For this review, take the finished solid that the model builds, in its own axes (mm). A direction names the side the tool comes from. Coordinates: 2 decimals unless noted, no trailing zeros. Write each loop counter-clockwise with the first axis right and the second up, starting at its lowest first coordinate (ties: lowest second). Pieces come first, ordered by that corner, then holes. Notation, with made-up numbers: (68, 68.5) -> (126, 68.5) arc R19 ccw to (126, 102.5) -> close; hole circle Ø2 at (0, 15.25). An arc over 180 degrees is marked (long way). One line per item, written item: value. Start each with the question number.
1) Machinability: for faces 1 (the flat face through (-44.45, 0, 0)), 2 (the cylindrical face through (42.22, 2.42, -0.1)), which of the approach directions +Z, -Z, +X, -X, +Y, -Y give a long, thin tool a straight path to every point of the face, cutting with its end or side? Answer none if there is none.
2) Add section A-A (z = -1). State the section outline as (x, y) points, and give its area (3 significant figures).
3) For probe 1 along Z at (x, y) = (39.5, 0.5); probe 2 along Z at (x, y) = (-35, 4.5); probe 3 along Y at (x, z) = (26.5, -3.5), list the stretches that pass through material, from the lowest coordinate up. Write a range as from..to.
4) Mouldability with a two-part tool opening along Z and no side actions: class faces 3 (the cylindrical face through (-0.62, -4.44, 4.54)), 4 (the cylindrical face through (0.62, -4.44, -4.54)), 5 (the cylindrical face through (47.306, -3.131, 0.223)) as released by +Z, released by -Z, zero draft, split by the parting line, or undercut.
5) For pin 1 Ø12 at (x, z) = (-21.5, -7) entering from -Y; pin 2 Ø1 at (x, z) = (-24, -4) entering from -Y; pin 3 Ø5 at (x, z) = (12.5, -6.5) entering from -Y, all flat-tipped, find the tip position at first contact; note any pin that passes through.
6) Add section C-C (y = -4). State the section outline as (x, z) points, and give its area (3 significant figures).
from build123d import *

# Parameters (mm, degrees)
F1_DEPTH = 6.35
F2_R     = 6.3499
F0_R     = 5.08
F3_DEPTH = 6.35


# Not quite as in the source:
# - a fillet or chamfer is up to 0.001 mm smaller than in the source, because OpenCascade refuses the exact size


with BuildPart() as f1:
    # F0 (on Front) → F1 (new body, symmetric)
    with BuildSketch(Plane.XZ):
        with BuildLine():
            Line((44.45, 6.35), (-44.45, 6.35))
            ThreePointArc((-44.45, 6.35), (-42.7945407024, 3.3649028089), (-42.221147458, 0))
            ThreePointArc((-42.221147458, 0), (-42.7945407024, -3.3649028089), (-44.45, -6.35))
            Line((-44.45, -6.35), (44.45, -6.35))
            ThreePointArc((44.45, -6.35), (42.221147458, 0), (44.45, 6.35))
        make_face()
        with BuildLine():
            ThreePointArc((-42.221147458, 0), (-42.7945407024, 3.3649028089), (-44.45, 6.35))
            Line((-44.45, 6.35), (-44.45, -6.35))
            ThreePointArc((-44.45, -6.35), (-42.7945407024, -3.3649028089), (-42.221147458, 0))
        make_face()
    extrude(amount=F1_DEPTH, both=True)

    # F2 (radius 6.35 in the source; OpenCascade refuses exactly that, so slightly less here)
    f2_edges = [f1.edges().sort_by_distance(p)[0] for p in [
        (0, -6.35, 6.35),
        (0, 6.35, 6.35),
        (0, -6.35, -6.35),
        (0, 6.35, -6.35),
    ]]
    fillet(f2_edges, radius=F2_R)

    # F0 (on Front) → F3 (join)
    with BuildSketch(Plane.XZ):
        with BuildLine():
            ThreePointArc((62.541147458, 0), (55.7460502669, 9.5866067556), (44.45, 6.35))
            Line((44.45, 6.35), (44.45, -6.35))
            ThreePointArc((44.45, -6.35), (55.7460502669, -9.5866067556), (62.541147458, 0))
        make_face()
        with Locations((52.381147458, 0)):
            Circle(F0_R, mode=Mode.SUBTRACT)
        with BuildLine():
            Line((44.45, -6.35), (44.45, 6.35))
            ThreePointArc((44.45, 6.35), (42.221147458, 0), (44.45, -6.35))
        make_face()
    extrude(amount=F3_DEPTH)


solid = f1.part
Numbers:
1. face 1: +Z, -Z, -X, +Y, -Y
1. face 2: +X, +Y
2. outline: (-44.45, -6.27) -> (42.27, -6.27) -> (42.27, -6.35) -> (47.4, -6.35) -> (47.4, 0) -> (42.27, 0) -> (42.27, 6.27) -> (-44.45, 6.27) -> close; (57.36, -6.35) -> (62.49, -6.35) -> (62.49, 0) -> (57.36, 0) -> close
2. area: 1,150 mm²
3. probe 1: -6.33..6.33
3. probe 2: -4.48..4.48
3. probe 3: -5.3..5.3
4. face 3: released by +Z
4. face 4: released by -Z
4. face 5: undercut
5. pin 1: y = -6.27
5. pin 2: y = -5.3
5. pin 3: y = -4.93
6. outline: (-44.45, -4.93) -> (43.5, -4.93) arc R10.16 ccw (long way) to (43.5, 4.93) -> (-44.45, 4.93) -> close; hole circle Ø10.16 at (52.38, 0)
6. area: 1,100 mm²
